Read the model definition and answer for the solid it produces. Units are mm, in the model's axes. Round coordinates to 2 decimals unless told otherwise and drop trailing zeros. Loops run counter-clockwise (first coordinate to the right, second up) from the corner with the lowest first, then second, coordinate; pieces in that order, holes last. Notation, with made-up numbers: (69.5, 30) - (82.5, 30) arc R19 ccw to (82.5, 53) - close; hole circle Ø8 at (-23, -8). An arc over 180 degrees is marked (long way). Use CSV: the item, a comma, the result in double quotes. Start each with the question number.
1. Consider line 1 along Y through (x, z) = (100, 1.85); line 2 along X through (y, z) = (48, 1); line 3 along X through (y, z) = (52, 0.55). Determine where each line is inside the solid, lowest interval first.
2. Find section A-A (x = 100). Give the vertices of the cut face in (y, z).
3. Given pin 1 Ø4 at (x, y) = (-30, 50) entering from +Z, flat-ended and moving along its own axis, determine where the tip first touches the part or whether it passes through.
4. Find section B-B (z = 1.6). Give the vertices of the cut face in (x, y).
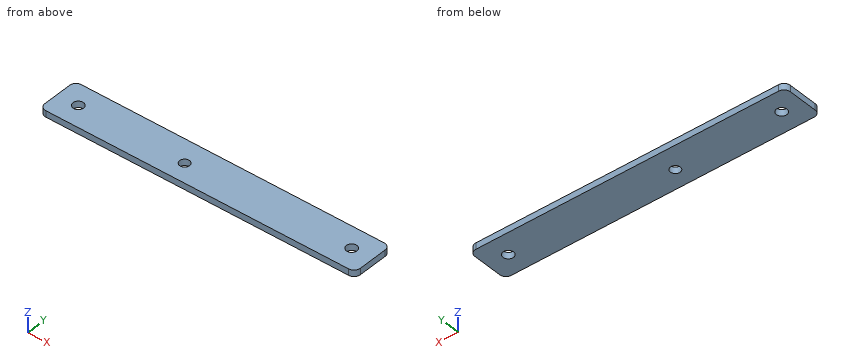
from build123d import *

# Parameters (mm, degrees)
SKETCH1_W           = 150
SKETCH1_H           = 20
SKETCH1_R           = 2.5
BOSS_EXTRUDE1_DEPTH = 3
FILLET1_R           = 3
SKETCH2_R           = 2.353501923
CUT_EXTRUDE1_DEPTH  = 108


with BuildPart() as part:
    # Sketch1 → Boss-Extrude1 (new body)
    with BuildSketch(Plane.XY):
        with Locations((35, 50)):
            Rectangle(SKETCH1_W, SKETCH1_H)
        with Locations((-30, 50)):
            Circle(SKETCH1_R, mode=Mode.SUBTRACT)
        with Locations((100, 50)):
            Circle(SKETCH1_R, mode=Mode.SUBTRACT)
    extrude(amount=BOSS_EXTRUDE1_DEPTH)

    # Fillet1
    fillet1_edges = [part.edges().sort_by_distance(p)[0] for p in [
        (110, 40, 1.5),
        (-40, 40, 1.5),
        (-40, 60, 1.5),
        (110, 60, 1.5),
    ]]
    fillet(fillet1_edges, radius=FILLET1_R)

    # Sketch2 → Cut-Extrude1 (cut)
    with BuildSketch(Plane.XY.offset(3)):
        with Locations((21.381283536, 49.013493537)):
            Circle(SKETCH2_R)
    extrude(amount=-CUT_EXTRUDE1_DEPTH, mode=Mode.SUBTRACT)


solid = part.part
Filled sheet:
1,line 1,"y = 40 to 47.5, 52.5 to 60"
1,line 2,"x = -40 to -31.5, -28.5 to 19.26, 23.51 to 98.5, 101.5 to 110"
1,line 3,"x = -40 to -31.5, -28.5 to 98.5, 101.5 to 110"
2,outline,"(40, 0) - (47.5, 0) - (47.5, 3) - (40, 3) - close; (52.5, 0) - (60, 0) - (60, 3) - (52.5, 3) - close"
3,pin 1,"passes through"
4,outline,"(-40, 43) arc R3 ccw to (-37, 40) - (107, 40) arc R3 ccw to (110, 43) - (110, 57) arc R3 ccw to (107, 60) - (-37, 60) arc R3 ccw to (-40, 57) - close; hole circle Ø5 at (-30, 50); hole circle Ø4.71 at (21.38, 49.01); hole circle Ø5 at (100, 50)"
